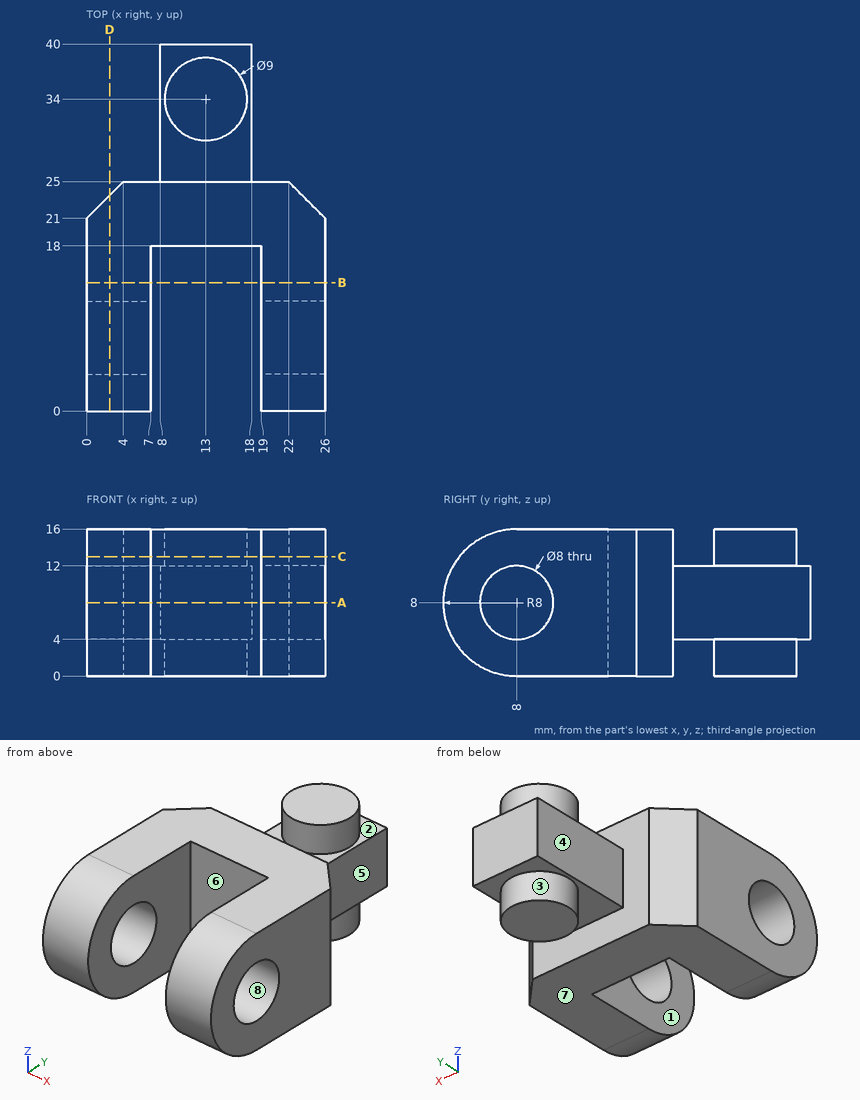
Here's the drawing with two shaded views (mm, measured from the low corner). I have some questions. A direction names the side the tool comes from. Give positions to 0.01 mm unless a question says otherwise; leave off trailing zeros. Order: outer loops, then holes, each group sorted by start corner. A loop starts at its lowest first (then second) coordinate and runs counter-clockwise, first axis right, second up.
Q1. We'd pull the mould along Y, two halves only. Please class the marked faces 6, 7 and 8: +Y half, -Y half, draft (parallel to the pull), parting line (faces both ways), or undercut.
Q2. Suppose I cut it at D-D, the plane x = 2.5. Write out the boundary of the cut face in (y, z).
Q3. I'm going to push flat-ended pins straight in: P1, Ø2.5, axis at y = 32.5, z = 7, coming from the +X side; P2, Ø2.5, axis at y = 35, z = 8, coming from the -X side. Where does each tip first touch, or does it pass through?
Q4. Suppose I cut it at B-B, the plane y = 14. Write out the boundary of the cut face in (x, z), and give its area (3 significant figures).
Q5. Suppose I cut it at A-A, the plane z = 8. Write out the boundary of the cut face in (x, y).
Q6. If I drill on line 1 along X through (y, z) = (12, 13.5); line 2 along Y through (x, z) = (7.25, 5.25); line 3 along Y through (x, z) = (21, 8), over which ranges is the centre line in solid material (lowest first)?
Q7. For the marked faces 1, 2, 3, 4 and 5, which set-ups out of +Z, -Z, +X, -X, +Y, -Y let a thin tool reach every point of the face, with its end or its side?
Q8. Suppose I cut it at C-C, the plane z = 13. Write out the boundary of the cut face in (x, y) (3 decimals).
Solution:
1. face 6: -Y half
1. face 7: draft
1. face 8: undercut
2. outline: (8, 0) - (23.5, 0) - (23.5, 16) - (8, 16) arc R8 ccw to start; hole circle Ø8 at (8, 8)
3. P1: stops at x = 18
3. P2: stops at x = 8
4. outline: (0, 0) - (7, 0) - (7, 16) - (0, 16) - close; (19, 0) - (26, 0) - (26, 16) - (19, 16) - close
4. area: 224 mm2
5. outline: (0, 0) - (7, 0) - (7, 4) - (0, 4) - close; (0, 12) - (7, 12) - (7, 18) - (19, 18) - (19, 12) - (26, 12) - (26, 21) - (22, 25) - (18, 25) - (18, 40) - (8, 40) - (8, 25) - (4, 25) - (0, 21) - close; (19, 0) - (26, 0) - (26, 4) - (19, 4) - close
6. line 1: x = 0 to 7, 19 to 26
6. line 2: y = 18 to 25
6. line 3: y = 0 to 4, 12 to 25
7. face 1: +Z, -Z, -Y
7. face 2: +Z
7. face 3: -Z
7. face 4: +Z, -Z, -X, +Y
7. face 5: +Z, -Z, +X, +Y
8. outline: (0, 1.755) - (7, 1.755) - (7, 18) - (19, 18) - (19, 1.755) - (26, 1.755) - (26, 21) - (22, 25) - (4, 25) - (0, 21) - close; circle Ø9 at (13, 34)
